from build123d import *

# Parameters (mm, degrees)
SKETCH_2_W          = 100
SKETCH_2_H          = 50
EXTRUDE_1_DEPTH     = 13
FILLET_1_R          = 10
SKETCH_3_R          = 10
CUT_EXTRUDE_1_DEPTH = 13
SKETCH_4_W          = 28.145361764
SKETCH_4_H          = 50
CUT_EXTRUDE_2_DEPTH = 13


with BuildPart() as part:
    # 草图2 → 凸台-拉伸1 (new body)
    with BuildSketch(Plane.XY):
        with Locations((-8.273923568, 5.39517388)):
            Rectangle(SKETCH_2_W, SKETCH_2_H)
    extrude(amount=EXTRUDE_1_DEPTH)

    # 圆角1
    fillet_1_edges = [part.edges().sort_by_distance(p)[0] for p in [
        (41.726076432, 30.39517388, 6.5),
    ]]
    fillet(fillet_1_edges, radius=FILLET_1_R)

    # 草图3 → 切除-拉伸1 (cut)
    with BuildSketch(Plane.XY.offset(13)):
        with Locations((8.064626437, 0)):
            Circle(SKETCH_3_R)
    extrude(amount=-CUT_EXTRUDE_1_DEPTH, mode=Mode.SUBTRACT)

    # 草图4 → 切除-拉伸2 (cut)
    with BuildSketch(Plane.XY.offset(13)):
        with Locations((-44.201242686, 5.39517388)):
            Rectangle(SKETCH_4_W, SKETCH_4_H)
    extrude(amount=-CUT_EXTRUDE_2_DEPTH, mode=Mode.SUBTRACT)


solid = part.part
The listing builds one solid part. Answer for the finished solid, in the listing's coordinates (mm). Coordinates: 2 decimals unless noted, no trailing zeros. Write each loop counter-clockwise with the first axis right and the second up, starting at its lowest first coordinate (ties: lowest second). Pieces come first, ordered by that corner, then holes. Notation, with made-up numbers: M 37,58 L 60,58 A12 cw 60,66 Z; hole C -34,55 d9. An arc over 180 degrees is marked long. Use one line per item in the form item = value.
Item 1: Given P1, Ø10, axis at x = 5, y = -1.5, coming from the +Z side, flat-ended and moving along its own axis, determine where the tip first touches the part or whether it passes through.
Model answer:
P1 = through
Item 2: Find section A-A, the plane y = 0. Give the vertices of the cut face in (x, z).
Model answer:
outline = M -30.13,0 L -1.94,0 L -1.94,13 L -30.13,13 Z; M 18.06,0 L 41.73,0 L 41.73,13 L 18.06,13 Z
Item 3: Find the intervals of material crossed by probe 1 along Y at (x, z) = (6, 6.25); probe 2 along Y at (x, z) = (12, 11.5); probe 3 along X at (y, z) = (4, 3.75), in increasing order.
Model answer:
probe_1 = -19.6 to -9.78, 9.78 to 30.4
probe_2 = -19.6 to -9.19, 9.19 to 30.4
probe_3 = -30.13 to -1.1, 17.23 to 41.73
Item 4: Find section B-B, the plane z = 8.5. Give the vertices of the cut face in (x, y).
Model answer:
outline = M -30.13,-19.6 L 41.73,-19.6 L 41.73,20.4 A10 ccw 31.73,30.4 L -30.13,30.4 Z; hole C 8.06,0 d20
Item 5: The mould has two halves that part along X. Classify faces 1 (the face through (5, -19.605, 6)), 2 (the face through (5.897, -9.762, 6.591)), 3 (the face through (-30.129, 5, 7)), 4 (the face through (38.87, 27.39, 6.59)): released by +X, released by -X, zero draft, split by the parting line, or undercut.
Model answer:
face_1 = zero draft
face_2 = undercut
face_3 = released by -X
face_4 = released by +X
Item 6: Find section D-D, the plane x = 37. Give the vertices of the cut face in (y, z).
Model answer:
outline = M -19.6,0 L 28.89,0 L 28.89,13 L -19.6,13 Z
Item 7: Find section C-C, the plane x = -1. Give the vertices of the cut face in (y, z).
Model answer:
outline = M -19.6,0 L -4.22,0 L -4.22,13 L -19.6,13 Z; M 4.22,0 L 30.4,0 L 30.4,13 L 4.22,13 Z
